Geometry check sheet. Reference: the model listing, model coordinates, mm. A direction names the side the tool comes from. Give positions to 0.01 mm unless a question says otherwise; leave off trailing zeros. Write each loop counter-clockwise with the first axis right and the second up, starting at its lowest first coordinate (ties: lowest second). Pieces come first, ordered by that corner, then holes.
(1) Cross-section at C-C (x = 39). Record the boundary of the cut face in (y, z).
(2) Cross-section at B-B (y = -4.5). Record the boundary of the cut face in (x, z), and give its area (3 significant figures).
(3) Cross-section at D-D (y = -44.5). Record the boundary of the cut face in (x, z).
(4) Thickness scan on line 1 along X through (y, z) = (-39, 35); line 2 along Y through (x, z) = (30.5, 0.5); line 3 along Z through (x, y) = (17, -44). Record the ranges inside material, lowest first.
(5) Mould release check, pull along Y, two halves, no side actions. Record for faces 4 (the flat face through (25, 1.53, -1)), 5 (the flat face through (50.851, -23, 14)), 6 (the flat face through (25, 2.8, 37)): +Y half, -Y half, draft (parallel to the pull), parting line (faces both ways), or undercut.
(6) Cross-section at A-A (z = 6.5). Record the boundary of the cut face in (x, y).
(7) Tool access check on faces 1 (the flat face through (25, -28, 64.059)), 2 (the flat face through (50, -25, -62.941)), 3 (the flat face through (25, -23, 62.789)). Record the directions out of +Z, -Z, +X, -X, +Y, -Y that give a thin tool (end or side, any length) a straight path to the whole face; none if there is none.
(8) Depth check by flat-ended pin: P1, Ø5, axis at x = 27.5, y = -14, coming from the +Z side; P2, Ø1, axis at x = 42.5, y = -35.5, coming from the -Z side. Enter the tip coordinate at first touch or a pass-through.
```python
from build123d import *

# Parameters (mm, degrees)
F0_W     = 50.8
F0_H     = 127
F1_DEPTH = 50.8508
F2_T     = -1.27
F3_W     = 50.8508
F3_H     = 10.889844
F4_DEPTH = 75.184


with BuildPart() as f1:
    # F0 (on Right) → F1 (new body)
    with BuildSketch(Plane.YZ):
        with Locations((-22.600227, 0.559007)):
            Rectangle(F0_W, F0_H)
    extrude(amount=F1_DEPTH)

    # F2
    f2_openings = [f1.faces().sort_by_distance(p)[0] for p in [
        (25.4254, -22.600227, -62.940993),
    ]]
    offset(amount=F2_T, openings=f2_openings)

    # F3 (on face) → F4 (join)
    with BuildSketch(Plane.XY.offset(64.059007)):
        with Locations((25.4254, -2.645149)):
            Rectangle(F3_W, F3_H)
    extrude(amount=F4_DEPTH)


solid = f1.part
```
Reply:
1. outline: (-48, -62.94) - (-46.73, -62.94) - (-46.73, 62.79) - (1.53, 62.79) - (1.53, -62.94) - (2.8, -62.94) - (2.8, 139.24) - (-8.09, 139.24) - (-8.09, 64.06) - (-48, 64.06) - close
2. outline: (0, -62.94) - (1.27, -62.94) - (1.27, 62.79) - (49.58, 62.79) - (49.58, -62.94) - (50.85, -62.94) - (50.85, 139.24) - (0, 139.24) - close
2. area: 4,210 mm2
3. outline: (0, -62.94) - (1.27, -62.94) - (1.27, 62.79) - (49.58, 62.79) - (49.58, -62.94) - (50.85, -62.94) - (50.85, 64.06) - (0, 64.06) - close
4. line 1: x = 0 to 1.27, 49.58 to 50.85
4. line 2: y = -48 to -46.73, 1.53 to 2.8
4. line 3: z = 62.79 to 64.06
5. face 4: undercut
5. face 5: draft
5. face 6: +Y half
6. outline: (0, -48) - (50.85, -48) - (50.85, 2.8) - (0, 2.8) - close; hole (1.27, -46.73) - (49.58, -46.73) - (49.58, 1.53) - (1.27, 1.53) - close
7. face 1: +Z, +X, -X, -Y
7. face 2: -Z, +X, -X, +Y, -Y
7. face 3: -Z
8. P1: stops at z = 64.06
8. P2: stops at z = 62.79
